Design review of the part shown in the three views and the two pictorial views. Dimensions are in mm from the part's minimum x, y and z. A direction names the side the tool comes from. Coordinates: 2 decimals unless noted, no trailing zeros. Write each loop counter-clockwise with the first axis right and the second up, starting at its lowest first coordinate (ties: lowest second). Pieces come first, ordered by that corner, then holes. Notation, with made-up numbers: (35.5, 89) - (57.5, 89) arc R9 ccw to (57.5, 106) - close; hole circle Ø8 at (50, -15). An arc over 180 degrees is marked (long way). Return JSON: item names as keys, results as strings. Group by question number.
(1) We need section C-C on x = 16. State the section outline as (y, z) points, then the cut area to 3 significant figures.
(2) For pin 1 Ø3.5 at (x, z) = (30, 2) entering from -Y; pin 2 Ø8 at (y, z) = (3.5, 17) entering from +X; pin 3 Ø12 at (y, z) = (2.5, 6) entering from -X, all flat-tipped, find the tip position at first contact; note any pin that passes through.
(3) We need section B-B on z = 16. State the section outline as (x, y) points.
(4) We need section A-A on z = 2. State the section outline as (x, y) points.
(5) Tool access review of the marked faces 1 and 2: name each direction out of +Z, -Z, +X, -X, +Y, -Y from which nothing blocks a thin tool from reaching the whole face with its end or side.
(6) To check wall thickness, follow L1, parallel to Z at x = 30, y = 22.8; L2, parallel to Y at x = 23.5, z = 14; L3, parallel to X at y = 6, z = 22. State the ranges of each line that lie inside material, in increasing order. Write a range as from..to.
(7) We need section D-D on y = 6.25. State the section outline as (x, z) points.
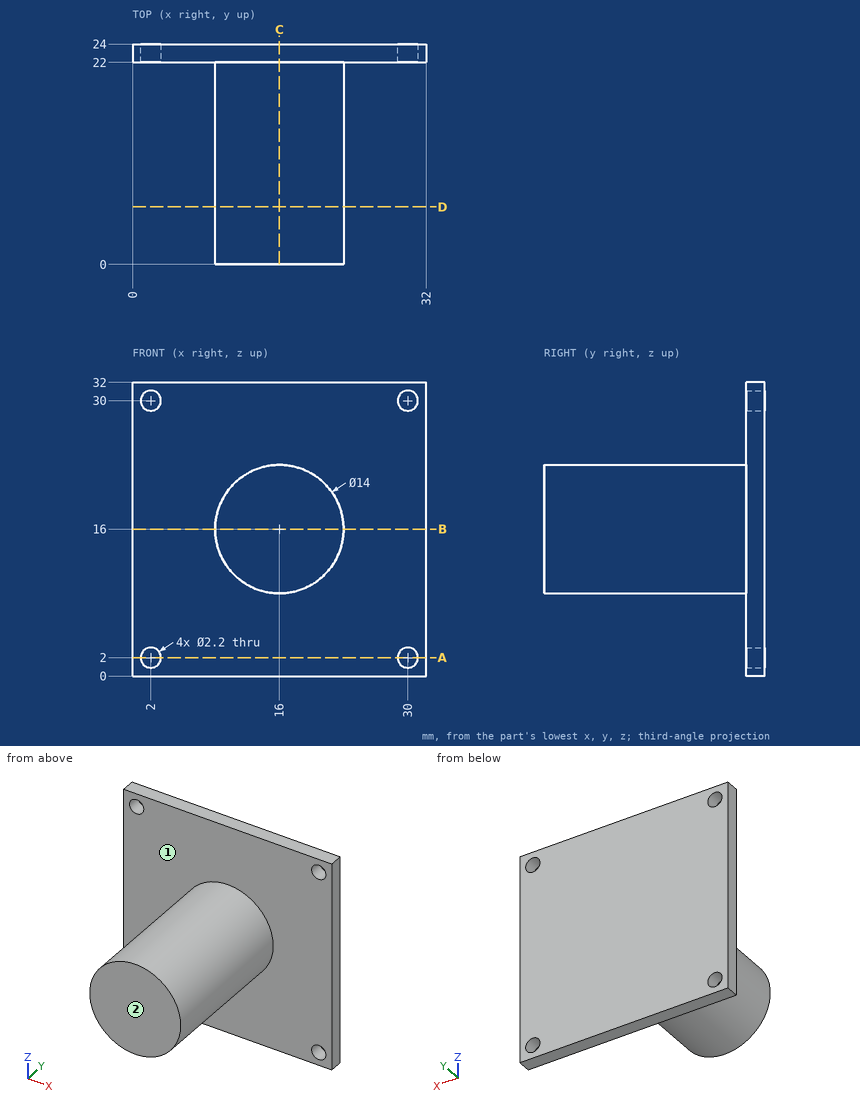
Ans:
{
 "1": {"outline": "(0, 9) - (22, 9) - (22, 0) - (24, 0) - (24, 32) - (22, 32) - (22, 23) - (0, 23) - close", "area": "372 mm²"},
 "2": {"pin 1": "y = 22", "pin 2": "x = 23", "pin 3": "x = 10.26"},
 "3": {"outline": "(0, 22) - (9, 22) - (9, 0) - (23, 0) - (23, 22) - (32, 22) - (32, 24) - (0, 24) - close"},
 "4": {"outline": "(0, 22) - (0.9, 22) - (0.9, 24) - (0, 24) - close; (3.1, 22) - (28.9, 22) - (28.9, 24) - (3.1, 24) - close; (31.1, 22) - (32, 22) - (32, 24) - (31.1, 24) - close"},
 "5": {"face 1": "-Y", "face 2": "+Z, -Z, +X, -X, -Y"},
 "6": {"L1": "0..0.9, 3.1..28.9, 31.1..32", "L2": "22..24", "L3": "12.39..19.61"},
 "7": {"outline": "circle Ø14 at (16, 16)"}
}
